Could you check a few things on this model? Use its own coordinates, in mm. Give positions to 0.01 mm unless a question says otherwise; leave off trailing zeros. Loops run counter-clockwise (first coordinate to the right, second up) from the corner with the lowest first, then second, coordinate; pieces in that order, holes last. Notation, with made-up numbers: (-13.5, 87.5) - (34.5, 87.5) arc R16 cw to (34.5, 117.5) - close; hole circle Ø5 at (61.25, -37.5). An arc over 180 degrees is marked (long way). Write each question's results on one line, items separated by ' | '. Start each with the question number.
(1) For pin 1 (1.5 mm diameter, centred on y = 1, z = -122, fed in from +X); pin 2 (3 mm diameter, centred on x = 54.5, y = 5, fed in from +Z); pin 3 (3 mm diameter, centred on x = 225, y = 3.5, fed in from -Z); pin 4 (1.9 mm diameter, centred on y = 4.5, z = -302.5, fed in from -X), each with a flat end and sliding along its axis, tell me the tip position at first contact or that it passes through.
(2) I need wall thicknesses on line 1 (Z direction, x = 180.5, y = 4.5); line 2 (X direction, y = 5.5, z = -51.5). Which ranges of each line are inside material? Lowest first, please.
(3) Suppose I cut it at A-A (x = 229.5). Please give me the cut outline in (y, z).
(4) Suppose I cut it at B-B (z = -79). Please give me the cut outline in (x, y).
from build123d import *

# Parameters (mm, degrees)
BOSS_EXTRUDE1_DEPTH = 6.35


with BuildPart() as part:
    # Sketch2 → Boss-Extrude1 (new body)
    with BuildSketch(Plane(origin=(0, 0, 0), x_dir=(1, 0, 0), z_dir=(0, 1, 0))):
        Polygon((0, 0), (152.4, 152.4), (0, 152.4), (0, 127), (6.35, 127), (6.35, 101.6), (0, 101.6), (0, 82.55), (6.35, 82.55), (6.35, 44.45), (0, 44.45), align=None)
        Polygon((127, 0), (152.4, 0), (152.4, 152.4), (0, 0), (44.45, 0), (44.45, 6.35), (82.55, 6.35), (82.55, 0), (101.6, 0), (101.6, 6.35), (127, 6.35), align=None)
        Polygon((152.4, 152.4), (152.4, 0), (177.8, 0), (177.8, 6.35), (203.2, 6.35), (203.2, 0), (222.25, 0), (222.25, 6.35), (260.35, 6.35), (260.35, 0), (304.8, 0), (304.8, 44.45), (298.45, 44.45), (298.45, 82.55), (304.8, 82.55), (304.8, 101.6), (298.45, 101.6), (298.45, 127), (304.8, 127), (304.8, 152.4), align=None)
        Polygon((304.8, 304.8), (152.4, 152.4), (304.8, 152.4), (304.8, 177.8), (298.45, 177.8), (298.45, 203.2), (304.8, 203.2), (304.8, 222.25), (298.45, 222.25), (298.45, 260.35), (304.8, 260.35), align=None)
        Polygon((152.4, 304.8), (152.4, 152.4), (304.8, 304.8), (260.35, 304.8), (260.35, 298.45), (222.25, 298.45), (222.25, 304.8), (203.2, 304.8), (203.2, 298.45), (177.8, 298.45), (177.8, 304.8), align=None)
        Polygon((0, 152.4), (152.4, 152.4), (152.4, 304.8), (127, 304.8), (127, 298.45), (101.6, 298.45), (101.6, 304.8), (82.55, 304.8), (82.55, 298.45), (44.45, 298.45), (44.45, 304.8), (0, 304.8), (0, 260.35), (6.35, 260.35), (6.35, 222.25), (0, 222.25), (0, 203.2), (6.35, 203.2), (6.35, 177.8), (0, 177.8), align=None)
    extrude(amount=BOSS_EXTRUDE1_DEPTH)


solid = part.part
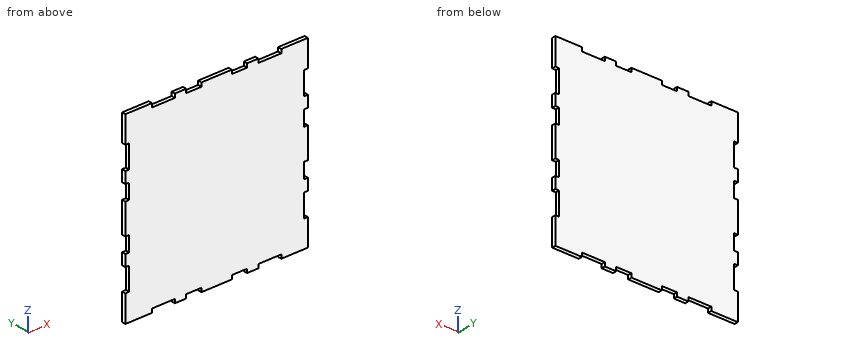
Output values:
1) pin 1: x = 298.45 | pin 2: z = -6.35 | pin 3: z = -298.45 | pin 4: x = 0
2) line 1: -298.45 to -6.35 | line 2: 6.35 to 298.45
3) outline: (0, -298.45) - (6.35, -298.45) - (6.35, -6.35) - (0, -6.35) - close
4) outline: (6.35, 0) - (298.45, 0) - (298.45, 6.35) - (6.35, 6.35) - close
